Work out the finished part from the listing and answer in its coordinate system (mm). Give positions to 0.01 mm unless a question says otherwise; leave off trailing zeros. Loops run counter-clockwise (first coordinate to the right, second up) from the corner with the lowest first, then second, coordinate; pieces in that order, holes last.
```python
from build123d import *

# Parameters (mm, degrees)
BOSS_EXTRUDE1_DEPTH      = 33.25
BOSS_EXTRUDE1_DEPTH_BACK = 33.25
SKETCH1_W                = 66.5
SKETCH1_H                = 66.5


with BuildPart() as part:
    # Sketch1 → Boss-Extrude1 (new, two sides: drawn at the far end of the back side and taken through both)
    with BuildSketch(Plane(origin=(0, 0, 0), x_dir=(1, 0, 0), z_dir=(0, 1, 0)).offset(-BOSS_EXTRUDE1_DEPTH_BACK)):
        Rectangle(SKETCH1_W, SKETCH1_H)
    extrude(amount=BOSS_EXTRUDE1_DEPTH + BOSS_EXTRUDE1_DEPTH_BACK)

    # Sketch2 → Cut-Revolve1 (revolve, cut)
    with BuildSketch(Plane(origin=(0, 0, 0), x_dir=(1, 0, 0), z_dir=(0, 1, 0))):
        with BuildLine():
            Line((-11.083333333, 0), (11.083333333, 0))
            ThreePointArc((11.083333333, 0), (0, 11.083333333), (-11.083333333, 0))
        make_face()
    revolve(axis=Axis((-11.083333333, 0, 0), (1, 0, 0)), mode=Mode.SUBTRACT)


solid = part.part
```
Q1. Section B-B on x = -1 is taken. Give the vertices of the cut face in (y, z), plus the area to 3 significant figures.
Q2. Section A-A on y = -9 is taken. Give the vertices of the cut face in (x, z).
Q3. Consider line 1 along Y through (x, z) = (10, -0.5); line 2 along Y through (x, z) = (-7, -3). Determine where each line is inside the solid, lowest interval first.
Check result:
1. outline: (-33.25, -33.25) - (33.25, -33.25) - (33.25, 33.25) - (-33.25, 33.25) - close; hole circle Ø22.08 at (0, 0)
1. area: 4,040 mm2
2. outline: (-33.25, -33.25) - (33.25, -33.25) - (33.25, 33.25) - (-33.25, 33.25) - close; hole circle Ø12.94 at (0, 0)
3. line 1: y = -33.25 to -4.75, 4.75 to 33.25
3. line 2: y = -33.25 to -8.05, 8.05 to 33.25
